from build123d import *

# Parameters (mm, degrees)
CYLINDER_R     = 3.9878
CYLINDER_DEPTH = 25.4
BOX001_W       = 50.8
BOX001_H       = 19.05
BOX001_DEPTH   = 3.175
BOX002_W       = 10.0076
BOX002_H       = 19.05
BOX002_DEPTH   = 6.35
BOX_W          = 50.8
BOX_H          = 19.05
BOX_DEPTH      = 3.175


with BuildPart() as cylinder:
    # Cylinder → Cylinder (new body)
    with BuildSketch(Plane(origin=(41.275, 9.525, -7.62), x_dir=(1, 0, 0), z_dir=(0, 0, 1))):
        Circle(CYLINDER_R)
    extrude(amount=CYLINDER_DEPTH)


with BuildPart() as cube001:
    # Box001 → Box001 (new body)
    with BuildSketch(Plane.XY.offset(-1.422)):
        with Locations((25.4, 9.525)):
            Rectangle(BOX001_W, BOX001_H)
    extrude(amount=BOX001_DEPTH)


with BuildPart() as cube002:
    # Box002 → Box002 (new body)
    with BuildSketch(Plane.XY.offset(1.676)):
        with Locations((5.0038, 9.525)):
            Rectangle(BOX002_W, BOX002_H)
    extrude(amount=BOX002_DEPTH)


with BuildPart() as cut:
    # Box → Box (new body)
    with BuildSketch(Plane.XY.offset(8.026)):
        with Locations((25.4, 9.525)):
            Rectangle(BOX_W, BOX_H)
    extrude(amount=BOX_DEPTH)

    # Fusion: union Cube001, Cube002
    add(cube001.part)
    add(cube002.part)

    # Cut: cut Cylinder
    add(cylinder.part, mode=Mode.SUBTRACT)


solid = cut.part
Read the model definition and answer for the solid it produces. Units are mm, in the model's axes. A direction names the side the tool comes from. Coordinates: 2 decimals unless noted, no trailing zeros. Order: outer loops, then holes, each group sorted by start corner. A loop starts at its lowest first (then second) coordinate and runs counter-clockwise, first axis right, second up. Notation, with made-up numbers: (-31.75, 66) - (18.25, 66) arc R17 cw to (18.25, 98) - close; hole circle Ø9 at (77, 37). An arc over 180 degrees is marked (long way). Use one line per item in the form item = value.
(1) Given pin 1 Ø1.9 at (y, z) = (5, 3.5) entering from +X, flat-ended and moving along its own axis, determine where the tip first touches the part or whether it passes through.
Computed values:
pin_1 = 10.01
(2) Which of the six approach directions +Z, -Z, +X, -X, +Y, -Y give full straight-line access (tool end or side, diameter ignored) to faces 5 (the face through (30, 10, 8.026)), 6 (the face through (25, 10, -1.422))?
Computed values:
face_5 = +X, +Y, -Y
face_6 = -Z, +X, -X, +Y, -Y
(3) Straight lines are drawn through the part: L1, parallel to Z at x = 41, y = 2.75; L2, parallel to X at y = 17.25, z = 2.25; L3, parallel to X at y = 9, z = 8.75. For each, find the intervals that lie inside material, in ascending order.
Computed values:
L1 = -1.42 to 1.75, 8.03 to 11.2
L2 = 0 to 10.01
L3 = 0 to 37.32, 45.23 to 50.8
(4) Section B-B, the plane y = 11.25 is taken. Give the vertices of the cut face in (x, z), then the cut area to 3 significant figures.
Computed values:
outline = (0, -1.42) - (37.68, -1.42) - (37.68, 1.75) - (10.01, 1.75) - (10.01, 8.03) - (37.68, 8.03) - (37.68, 11.2) - (0, 11.2) - close; (44.87, -1.42) - (50.8, -1.42) - (50.8, 1.75) - (44.87, 1.75) - close; (44.87, 8.03) - (50.8, 8.03) - (50.8, 11.2) - (44.87, 11.2) - close
area = 340 mm²
(5) Section C-C, the plane x = 41.5 is taken. Give the vertices of the cut face in (y, z), then the cut area to 3 significant figures.
Computed values:
outline = (0, -1.42) - (5.54, -1.42) - (5.54, 1.75) - (0, 1.75) - close; (0, 8.03) - (5.54, 8.03) - (5.54, 11.2) - (0, 11.2) - close; (13.51, -1.42) - (19.05, -1.42) - (19.05, 1.75) - (13.51, 1.75) - close; (13.51, 8.03) - (19.05, 8.03) - (19.05, 11.2) - (13.51, 11.2) - close
area = 70.4 mm²
(6) For a pull along Y with two mould halves and no side action, classify faces 1 (the face through (19, 19.05, 1)), 2 (the face through (19, 0, 1)), 3 (the face through (44.96, 8, 9.59)), 4 (the face through (0, 9, 5)) as pulls with the +Y half, pulls with the -Y half, needs draft (parallel to the pull), parting line crosses it, or undercut.
Computed values:
face_1 = pulls with the +Y half
face_2 = pulls with the -Y half
face_3 = undercut
face_4 = needs draft
(7) Section D-D, the plane y = 15 is taken. Give the vertices of the cut face in (x, z), then the cut area to 3 significant figures.
Computed values:
outline = (0, -1.42) - (50.8, -1.42) - (50.8, 1.75) - (10.01, 1.75) - (10.01, 8.03) - (50.8, 8.03) - (50.8, 11.2) - (0, 11.2) - close
area = 385 mm²
(8) Section A-A, the plane x = 47 is taken. Give the vertices of the cut face in (y, z).
Computed values:
outline = (0, -1.42) - (19.05, -1.42) - (19.05, 1.75) - (0, 1.75) - close; (0, 8.03) - (19.05, 8.03) - (19.05, 11.2) - (0, 11.2) - close
